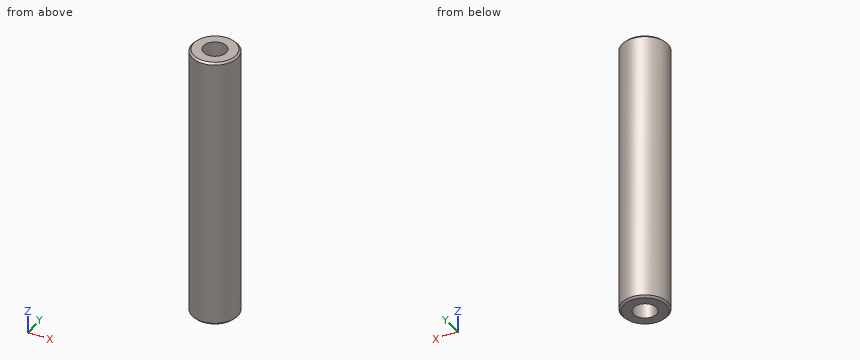
```python
from build123d import *

# Parameters (mm, degrees)
SKETCH_1_W     = 30
SKETCH_1_H     = 2.5
CHAMFER_1_SIZE = 0.2


with BuildPart() as part:
    # 草图1 → 旋转1 (revolve)
    with BuildSketch(Plane(origin=(0, 0, 0), x_dir=(0, 0, -1), z_dir=(1, 0, 0)), mode=Mode.PRIVATE) as revolve_1_sk:
        with Locations((0, 1.25)):
            Rectangle(SKETCH_1_W, SKETCH_1_H)
    revolve(revolve_1_sk.sketch.rotate(Axis((0, 0, 15), (0, 0, -1)), 180), axis=Axis((0, 0, 15), (0, 0, -1)))

    # 草图3 → Hole Wizard 1 (revolve, cut)
    with BuildSketch(Plane(origin=(0, 0, 15), x_dir=(0, -1, 0), z_dir=(1, 0, 0))):
        Polygon((0, 0), (0, 14.251075774), (1.25, 13.5), (1.25, 0), align=None)
    hole_wizard_1 = revolve(axis=Axis((0, 0, 21.35), (0, 0, -1)), mode=Mode.SUBTRACT)

    # 镜向1: Hole Wizard 1 across plane
    add(hole_wizard_1.mirror(Plane.XY), mode=Mode.SUBTRACT)

    # 倒角1
    chamfer_1_edges = [part.edges().sort_by_distance(p)[0] for p in [
        (0, 2.5, -15),
        (0, 2.5, 15),
    ]]
    chamfer(chamfer_1_edges, length=CHAMFER_1_SIZE)


solid = part.part
```
Geometry: final body of the model. Coordinates: model frame, mm. Give positions to 0.01 mm unless a question says otherwise; leave off trailing zeros. Order: outer loops, then holes, each group sorted by start corner. A loop starts at its lowest first (then second) coordinate and runs counter-clockwise, first axis right, second up. Notation, with made-up numbers: M -25.75,6 L 5.25,6 A14 ccw 5.25,12 Z; hole C 40,53 d7. An arc over 180 degrees is marked long. Answer as CSV lines item,"result". Start each with the question number.
1) First-contact query: P1, Ø1.5, axis at x = 0, y = 0, coming from the -Z side. Flat tip, straight axial feed; report the tip coordinate or a pass-through.
2) Line query: line 1 (X direction, y = 0, z = -5.25); line 2 (Y direction, x = -0.9, z = 12.75); line 3 (Y direction, x = -0.55, z = -6). Output: solid intervals per line, ascending. Write a range as from..to.
3) Cut plane A-A (z = -2.5). Output: boundary loops of the cut face in (x, y), then the cut area to 3 significant figures.
Findings below:
1,P1,"stops at z = -1.2"
2,line 1,"x = -2.5..-1.25, 1.25..2.5"
2,line 2,"y = -2.33..-0.87, 0.87..2.33"
2,line 3,"y = -2.44..-1.12, 1.12..2.44"
3,outline,"C 0,0 d5; hole C 0,0 d2.5"
3,area,"14.7 mm²"
